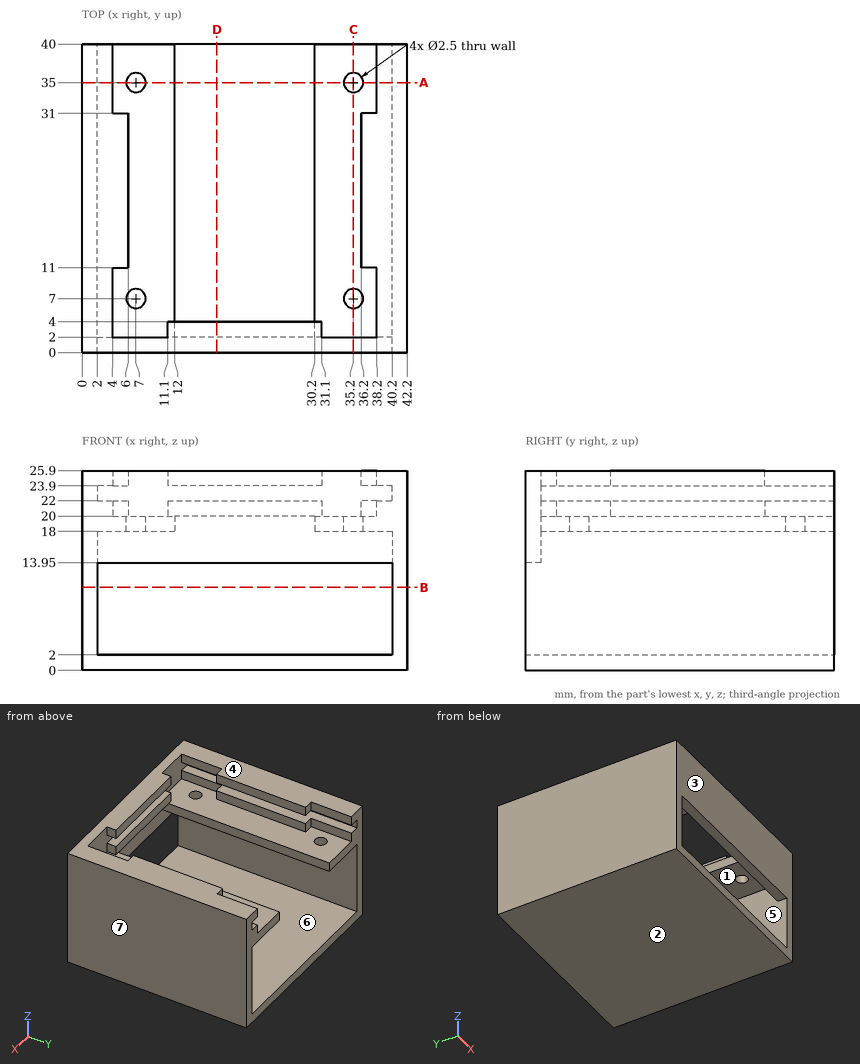
Study the drawing (mm; zero at the part's minimum x, y, z) and answer. A direction names the side the tool comes from. Give positions to 0.01 mm unless a question says otherwise; leave off trailing zeros. Write each loop counter-clockwise with the first axis right and the second up, starting at its lowest first coordinate (ties: lowest second). Pieces come first, ordered by that corner, then holes. Notation, with made-up numbers: (20.5, 72.25) -> (51.5, 72.25) arc R4 ccw to (51.5, 79.25) -> close; hole circle Ø7 at (-38.5, -32). An arc over 180 degrees is marked (long way). Answer in a Markdown table with one row per item.
1) Straight lines are drawn through the part: line 1 (Y direction, x = 35.2, z = 18.95); line 2 (Z direction, x = 4.5, y = 23.5); line 3 (Z direction, x = 25.5, y = 3.5). For each, find the intervals that lie inside material, in ascending order. Write a range as [from, to].
Results list:
| item | result |
|---|---|
| line 1 | [0, 5.75], [8.25, 33.75], [36.25, 40] |
| line 2 | [0, 2], [18, 22], [23.9, 25.9] |
| line 3 | [0, 2], [20, 22], [23.9, 25.9] |
2) Section A-A on y = 35 is taken. Count the separate pieces of the cut face and the enclosed holes in it, plus the area to 3 significant figures.
Results list:
| item | result |
|---|---|
| separate pieces | 3 |
| enclosed holes | 0 |
| area | 226 mm^2 |
3) A tool of negligible diameter and unlimited length cuts with its end or side. For the marked faces 5, 6 and 7, from which of +Z, -Z, +X, -X, +Y, -Y can it reach the whole face along a straight path? Write none if from no direction.
Results list:
| item | result |
|---|---|
| face 5 | +Y |
| face 6 | +Y, -Y |
| face 7 | +Z, -Z, +X, +Y, -Y |
4) Section B-B on z = 10.75 is taken. Give the vertices of the cut face in (x, y), plus the area to 3 significant figures.
Results list:
| item | result |
|---|---|
| outline | (0, 0) -> (2, 0) -> (2, 40) -> (0, 40) -> close; (40.2, 0) -> (42.2, 0) -> (42.2, 40) -> (40.2, 40) -> close |
| area | 160 mm^2 |
5) Section D-D on x = 17.5 is taken. Give the vertices of the cut face in (y, z).
Results list:
| item | result |
|---|---|
| outline | (0, 0) -> (40, 0) -> (40, 2) -> (0, 2) -> close; (0, 13.95) -> (2, 13.95) -> (2, 20) -> (4, 20) -> (4, 22) -> (2, 22) -> (2, 23.9) -> (4, 23.9) -> (4, 25.9) -> (0, 25.9) -> close |
6) Each of these flat-tipped pins is pushed along its axis until it touches: pin 1 Ø6.5 at (x, z) = (24, 22.5) entering from +Y; pin 2 Ø1 at (y, z) = (3, 21) entering from -X; pin 3 Ø6 at (x, y) = (24.5, 28) entering from +Z. Where does it stop, or does it pass through?
Results list:
| item | result |
|---|---|
| pin 1 | y = 4 |
| pin 2 | x = 0 |
| pin 3 | z = 2 |
7) Determine the mould class of the marked faces 1, 2, 3 and 4 for opening direction Z: released by +Z, released by -Z, zero draft, split by the parting line, or undercut.
Results list:
| item | result |
|---|---|
| face 1 | undercut |
| face 2 | released by -Z |
| face 3 | zero draft |
| face 4 | released by +Z |
8) Section C-C on x = 35.2 is taken. Give the vertices of the cut face in (y, z).
Results list:
| item | result |
|---|---|
| outline | (0, 0) -> (40, 0) -> (40, 2) -> (0, 2) -> close; (0, 13.95) -> (2, 13.95) -> (2, 18) -> (5.75, 18) -> (5.75, 20) -> (2, 20) -> (2, 25.9) -> (0, 25.9) -> close; (8.25, 18) -> (33.75, 18) -> (33.75, 20) -> (8.25, 20) -> close; (36.25, 18) -> (40, 18) -> (40, 20) -> (36.25, 20) -> close |
